Design review of the part built by this model. Coordinates are the model's own, in mm. A direction names the side the tool comes from. Round coordinates to 2 decimals unless told otherwise and drop trailing zeros. Loops run counter-clockwise (first coordinate to the right, second up) from the corner with the lowest first, then second, coordinate; pieces in that order, holes last. Notation, with made-up numbers: (-2, -36.5) -> (4, -36.5) arc R24 cw to (4, -24.5) -> close; hole circle Ø5 at (82, 9). An arc over 180 degrees is marked (long way). Answer as CSV lines item,"result". Start each with the question number.
(1) Take a section at B-B, the plane y = 4.4. Write out the cut boundary in (x, z), and give its area (3 significant figures).
(2) Machinability: for faces 1 (the face through (11, 2.54, -4)), 2 (the face through (5, 5.08, 4)), which of the approach directions +Z, -Z, +X, -X, +Y, -Y give a long, thin tool a straight path to every point of the face, cutting with its end or side? Answer none if there is none.
(3) For P1, Ø2, axis at x = 3.5, y = 1.5, coming from the -Z side; P2, Ø8, axis at x = 12.5, z = -3, coming from the +Y side; P3, Ø1.5, axis at x = 5, y = 1, coming from the +Z side, all flat-tipped, find the tip position at first contact; note any pin that passes through.
(4) Draft analysis for pull direction Z (two halves, no side actions). For faces 3 (the face through (7.61, 3.79, 3.11)), 4 (the face through (9.21, 1.25, -4.8)), 5 (the face through (11, 0, -3)), state which applies: +Z half, -Z half, draft (parallel to the pull), parting line (faces both ways), or undercut.
(5) To check wall thickness, follow line 1 (Y direction, x = 6.25, z = -6.75); line 2 (Z direction, x = 4.75, y = 0.95); line 3 (Z direction, x = 7, y = 2.5). State the ranges of each line that lie inside material, in increasing order. Write a range as from..to.
(6) Take a section at C-C, the plane z = -9.75. Write out the cut boundary in (x, y).
(7) Take a section at D-D, the plane y = 0.55. Write out the cut boundary in (x, z) (1 decimal), and give its area (3 significant figures).
(8) Take a section at A-A, the plane x = 6.5. Write out the cut boundary in (y, z), and give its area (3 significant figures).
Autodesk Inventor part; units mm, degrees
ref_plane "YZ Plane" through (0, 0, 0) normal (1, 0, 0) x (0, 1, 0)
ref_plane "XZ Plane" through (0, 0, 0) normal (0, 1, 0) x (-1, 0, 0)
ref_plane "XY Plane" through (0, 0, 0) normal (0, 0, 1) x (1, 0, 0)
sketch "Sketch1" plane through (0, 0, 0) normal (0, 1, 0) x (-1, 0, 0)
  line L0 (6.5186, 9.6083) -> (7.4793, 6.9251)
  line L1 (9.9904, -0.6602) -> (10.9974, -3.3263)
  line L2 (6.9989, 8.2667) -> (-2.8141, 4.7803)
  line L3 (10.4939, -1.9933) -> (0.6808, -5.4797)
  circle A0 centre (-12.8288, -4.5578) radius 1.5875
  circle A1 centre (-12.8288, -4.5578) radius 3.3389
  line L4 (-2.8141, 4.7803) -> (-12.8288, -4.5578)
  line L5 (-12.8288, -4.5578) -> (0.6808, -5.4797)
  line L6 (-2.8141, 4.7803) -> (-15.056, 0.431)
  line L7 (-12.8288, -4.5578) -> (-14.6522, 0.5745)
  line L8 (-14.6522, 0.5745) -> (-2.8141, 4.7803)
  line L9 (-12.8288, -4.5578) -> (-10.8725, -10.064)
  line L10 (0.6808, -5.4797) -> (-10.8725, -10.064)
  line L11 (10.4939, -1.9933) -> (11.3914, -4.3694)
  line L12 (11.3914, -4.3694) -> (9.5964, 0.3829)
  line L13 (9.5964, 0.3829) -> (-15.056, -8.4497)
  line L14 (-12.8288, -4.5578) -> (-15.975, -5.6756)
  line L15 (-15.9757, -5.6736) -> (-13.4484, -12.787)
  line L16 (-13.4484, -12.787) -> (-12.5471, -15.637)
  line L17 (11.3914, -4.3694) -> (-13.0447, -14.0634)
  line L18 (-15.9757, -5.6736) -> (-19.6824, 6.0465)
  line L19 (6.9989, 8.2667) -> (7.8493, 5.8733)
  line L20 (7.8493, 5.8733) -> (6.1486, 10.6602)
  line L21 (6.1486, 10.6602) -> (-18.3849, 1.9439)
  line L22 (7.8493, 5.8733) -> (-16.8521, -2.9027)
  line L23 (-2.8141, 4.7803) -> (0.6808, -5.4797)
  line L24 (-2.8141, 4.7803) -> (-3.6645, 7.1738)
  line L25 (0.6808, -5.4797) -> (1.6582, -8.2307)
  line L26 (-1.9951, 2.3758) -> (-16.8521, -2.9027)
  line L27 (-3.6645, 7.1738) -> (-18.3849, 1.9439)
  line L28 (-13.0447, -14.0634) -> (1.6582, -8.2307)
  line L29 (-0.1292, -3.1017) -> (-11.8537, -7.3024)
  line L30 (-0.1292, -3.1017) -> (1.6582, -8.2307)
  line L31 (-12.8288, -4.5578) -> (-9.6759, -3.4591)
  line L32 (-9.6759, -3.4591) -> (-6.8384, -11.6013)
  line L33 (-9.6759, -3.4591) -> (-12.2361, 4.1284)
  point P0 (0, 0)
  point P1 (-8.727, -6.1821)
  point P2 (-10.6118, -0.6856)
  point P3 (-16.045, -5.4546)
  point P4 (-15.9742, -5.6777)
  dimension "d0" = 10.414
  dimension "d1" = 10.414
  dimension "d2" = 12.2419
  dimension "d3" = 12.4297
  dimension "d4" = 5.1323
  dimension "d5" = 5.5062
  dimension "d6" = 13.6929
  dimension "d7" = 13.5096
  dimension "d8" = 2.54
  dimension "d9" = 5.08
  dimension "d10" = 2.54
  dimension "d11" = 5.08
sketch "Sketch2" plane through (0, 0, 0) normal (0, 1, 0) x (-1, 0, 0)
  point P0 (0, 0)
extrude "Extrusion1" add sketch "Sketch1" along normal blind 2.54 contours L18 L22 A1 | L23 L5 L13 | L10 L32 L13 L5 | L25 L17 L32 L10 | L22 L4 L23 | L32 L17 L16 L15 L13 A1 L9 L10 | L10 L9 A1 L13 L32 | L32 L13 A1 L5 | L5 A1 L32 | L22 L33 L6 L4 | L6 L33 L21 L24 | L5 A0 L31 A1 | A1 L13 L9 A0 L5 | L31 A0 L4 A1 | A1 L4 L33 | A1 L9 L13 | L4 A1 L22 L33 | L22 A1 L7 L6 L33 | L6 L7 A1 L22 L18 L21 L33 | A1 L13 L9 | L5 L31 A0 | A0 L9 L5 | L4 A0 L7 L22 A1 | L31 L4 A0 | L13 A1 L14 A0 L9 | L22 L7 A1 | L13 L15 A1 | A0 L14 L9 | L7 A0 L4 | L14 A0 L7 | L7 L22 A1 | L7 A0 L14 A1 L22
sketch "Sketch3" plane through (0, 2.54, 0) normal (0, 1, 0) x (1, 0, 0)
  line L0 (8.727, 6.1821) -> (6.8384, 11.6013)
  line L1 (13.0447, 14.0634) -> (-1.6582, 8.2307)
  line L2 (10.6118, 0.6856) -> (12.2361, -4.1284)
  line L3 (3.6645, -7.1738) -> (18.3849, -1.9439)
  line L4 (8.727, 6.1821) -> (9.6759, 3.4591)
  line L5 (9.6759, 3.4591) -> (10.6118, 0.6856)
  point P0 (0, 0)
sketch "Sketch4" plane through (0, 2.54, 0) normal (0, 1, 0) x (1, 0, 0)
  line L0 (2.8141, -4.7803) -> (3.6645, -7.1738)
  line L1 (1.9951, -2.3758) -> (3.6645, -7.1738)
  line L2 (3.6645, -7.1738) -> (8.4513, -5.4731)
  line L3 (3.6645, -7.1738) -> (18.3849, -1.9439)
  line L4 (8.4513, -5.4731) -> (6.7507, -0.6862)
  line L5 (10.6118, 0.6856) -> (1.9951, -2.3758)
  line L6 (-0.6808, 5.4797) -> (0.1292, 3.1017)
  line L7 (0.1292, 3.1017) -> (4.9115, 4.8151)
  line L8 (0.1292, 3.1017) -> (8.727, 6.1821)
  line L9 (4.9115, 4.8151) -> (3.0225, 10.0875)
  line L10 (13.0447, 14.0634) -> (-1.6582, 8.2307)
  line L11 (3.6645, -7.1738) -> (18.3849, -1.9439)
  line L12 (-1.6582, 8.2307) -> (-0.6808, 5.4797)
  line L13 (-0.6808, 5.4797) -> (-1.6582, 8.2307)
  point P0 (0, 0)
  dimension "d14" = 5.08
  dimension "d15" = 5.08
sketch "Sketch5" plane through (0, 2.54, 0) normal (0, 1, 0) x (1, 0, 0)
  point P0 (0, 0)
extrude "Extrusion2" add sketch "Sketch4" along normal blind 2.54
properties part number "filendholder"
The answers:
1,outline,"(-1.66, -8.23) -> (3.02, -10.09) -> (4.91, -4.82) -> (0.13, -3.1) -> (-0.68, -5.48) -> close; (2, 2.38) -> (6.75, 0.69) -> (8.45, 5.47) -> (3.66, 7.17) -> close"
1,area,"53.6 mm²"
2,face 1,"-Z, +X, +Y"
2,face 2,"+Z, -Z, +X, -X, +Y"
3,P1,"z = -10.67"
3,P2,"y = 2.54"
3,P3,"z = 6.97"
4,face 3,"-Z half"
4,face 4,"undercut"
4,face 5,"draft"
5,line 1,"0..2.54"
5,line 2,"-10.77..-4.76, 1.4..6.79"
5,line 3,"-11.67..-5.56, 0.6..5.99"
6,outline,"(2.17, 0) -> (14.53, 0) -> (14.53, 2.54) -> (3.14, 2.54) -> (3.14, 5.08) -> (2.17, 5.08) -> close"
7,outline,"(-1.7, -8.2) -> (13, -14.1) -> (13.4, -12.8) -> (16, -5.7) -> (18.4, 1.9) -> (3.7, 7.2) -> (2.8, 4.8) -> (2, 2.4) -> (10.6, -0.7) -> (9.7, -3.5) -> (8.7, -6.2) -> (0.1, -3.1) -> (-0.7, -5.5) -> close"
7,area,"208 mm²"
8,outline,"(0, -11.47) -> (2.54, -11.47) -> (2.54, -5.38) -> (0, -5.38) -> close; (0, 0.78) -> (5.08, 0.78) -> (5.08, 6.17) -> (0, 6.17) -> close"
8,area,"42.8 mm²"
